Autodesk Inventor part; units mm, degrees
ref_plane "YZ Plane" through (0, 0, 0) normal (1, 0, 0) x (0, 1, 0)
ref_plane "XZ Plane" through (0, 0, 0) normal (0, 1, 0) x (-1, 0, 0)
ref_plane "XY Plane" through (0, 0, 0) normal (0, 0, 1) x (1, 0, 0)
sketch "Sketch1" plane through (0, 0, 0) normal (0, 1, 0) x (-1, 0, 0)
  line L0 (22.352, 6.35) -> (-46.355, 6.35)
  line L1 (-46.355, 6.35) -> (-46.355, -6.35)
  line L2 (-46.355, -6.35) -> (22.352, -6.35)
  line L3 (22.352, -6.35) -> (22.352, 6.35)
  line L4 (-2.3114, -2.3114) -> (2.3114, -2.3114)
  line L5 (2.3114, -2.3114) -> (2.3114, 2.3114)
  line L6 (2.3114, 2.3114) -> (-2.3114, 2.3114)
  line L7 (-2.3114, 2.3114) -> (-2.3114, -2.3114)
  line L8 (-2.3114, -2.3114) -> (2.3114, 2.3114) construction
  line L9 (2.3114, -2.3114) -> (-2.3114, 2.3114) construction
  line L10 (-10.3886, 2.3114) -> (-15.0114, 2.3114)
  line L11 (-15.0114, 2.3114) -> (-15.0114, -2.3114)
  line L12 (-15.0114, -2.3114) -> (-10.3886, -2.3114)
  line L13 (-10.3886, -2.3114) -> (-10.3886, 2.3114)
  line L14 (-10.3886, 2.3114) -> (-15.0114, -2.3114) construction
  line L15 (-15.0114, 2.3114) -> (-10.3886, -2.3114) construction
  line L16 (-23.0886, 2.3114) -> (-27.7114, 2.3114)
  line L17 (-27.7114, 2.3114) -> (-27.7114, -2.3114)
  line L18 (-27.7114, -2.3114) -> (-23.0886, -2.3114)
  line L19 (-23.0886, -2.3114) -> (-23.0886, 2.3114)
  line L20 (-23.0886, 2.3114) -> (-27.7114, -2.3114) construction
  line L21 (-27.7114, 2.3114) -> (-23.0886, -2.3114) construction
  point P0 (0, 0)
  point P1 (-12.7, 0)
  point P2 (-25.4, 0)
  dimension "d0" = 68.707
  dimension "d1" = 12.7
  dimension "d2" = 4.6228
  dimension "d3" = 4.6228
  dimension "d4" = 4.6228
  dimension "d5" = 4.6228
  dimension "d6" = 12.7
  dimension "d7" = 12.7
  dimension "d8" = 6.35
  dimension "d9" = 22.352
extrude "Extrusion1" add sketch "Sketch1" along normal blind 1.1684
sketch "Sketch2" plane through (0, 1.1684, 0) normal (0, 1, 0) x (1, 0, 0)
  line L0 (-22.352, 6.35) -> (-22.352, -6.35)
  circle A0 centre (-16.002, 0) radius 4.0259
  point P0 (0, 0)
  dimension "d12" = 6.35
  dimension "d13" = 8.0518
extrude "Extrusion2" add sketch "Sketch2" along normal blind 6.8326
sketch "Sketch3" plane through (-16.002, 8.001, 0) normal (0, 1, 0) x (1, 0, 0)
  circle A0 centre (0, 0) radius 2.8575
  point P0 (16.002, 0)
  dimension "d16" = 5.715
extrude "Extrusion3" cut sketch "Sketch3" against normal blind 0.7874
sketch "Sketch4" plane through (0, 0, 0) normal (0, -1, 0) x (1, 0, 0)
  circle A0 centre (-16.002, 0) radius 2.8575
  circle A1 centre (-16.002, 0) radius 2.8575
  point P0 (0, 0)
extrude "Extrusion4" cut sketch "Sketch4" against normal blind 0.7874
sketch "Sketch5" plane through (-16.002, 7.2136, 0) normal (0, 1, 0) x (1, 0, 0)
  circle A0 centre (0, 0) radius 2.4511
  point P0 (16.002, 0)
  dimension "d21" = 4.9022
extrude "Extrusion5" cut sketch "Sketch5" against normal through all
sketch "Sketch6" plane through (0, 1.1684, 0) normal (0, 1, 0) x (1, 0, 0)
  line L0 (46.355, -6.35) -> (46.355, 6.35)
  circle A0 centre (40.005, 0) radius 4.0259
  point P0 (0, 0)
  dimension "d24" = 6.35
  dimension "d25" = 8.0518
extrude "Extrusion6" add sketch "Sketch6" along normal blind 6.8326
sketch "Sketch7" plane through (40.005, 8.001, 0) normal (0, 1, 0) x (1, 0, 0)
  circle A0 centre (0, 0) radius 2.8575
  point P0 (-40.005, 0)
  dimension "d28" = 5.715
extrude "Extrusion7" cut sketch "Sketch7" against normal blind 0.7874
sketch "Sketch8" plane through (0, 0, 0) normal (0, -1, 0) x (1, 0, 0)
  circle A0 centre (40.005, 0) radius 2.8575
  circle A1 centre (40.005, 0) radius 2.8575
  point P0 (0, 0)
extrude "Extrusion8" cut sketch "Sketch8" against normal blind 0.7874
sketch "Sketch9" plane through (40.005, 7.2136, 0) normal (0, 1, 0) x (1, 0, 0)
  circle A0 centre (0, 0) radius 2.4511
  point P0 (-40.005, 0)
  dimension "d33" = 4.9022
extrude "Extrusion9" cut sketch "Sketch9" against normal through all
properties part number "VexLegoMount"
The model under review builds one solid part; all positions refer to its coordinate system, in mm. A direction names the side the tool comes from. Round coordinates to 2 decimals unless told otherwise and drop trailing zeros. Loops run counter-clockwise (first coordinate to the right, second up) from the corner with the lowest first, then second, coordinate; pieces in that order, holes last. Notation, with made-up numbers: M 2,-14.75 L 11,-14.75 A31 cw 11,21.25 Z; hole C 49.5,56 d3. An arc over 180 degrees is marked long. Answer as CSV lines item,"result". Start each with the question number.
Item 1: Insertion check: P1, Ø2, axis at y = 6, z = -2, coming from the -X side; P2, Ø3, axis at y = 4.5, z = 3, coming from the -X side. Each pin has a flat end and moves straight along its axis. Give the tip position at first contact, or say it passes through.
Item 2: Mouldability with a two-part tool opening along X and no side actions: class faces 4 (the face through (42.73, 0.39, 0.86)), 5 (the face through (46.355, 1, 0)), 6 (the face through (12, 0, -3)) as released by +X, released by -X, zero draft, split by the parting line, or undercut.
Item 3: Consider section C-C (x = -8.5). Write out the cut boundary in (y, z), then the cut area to 3 significant figures.
Item 4: Consider section D-D (z = 5.25). Write out the cut boundary in (x, y) (3 decimals).
Item 5: Wall thickness on line 1 (X direction, y = 3.25, z = 0.25); line 2 (X direction, y = 4, z = 0); line 3 (Z direction, x = -16, y = 4.75): over which ranges is each line inside the solid? List them lowest first. Write a range as [from, to].
Item 6: For faces 1 (the face through (35.983, 4.537, 0.177)), 2 (the face through (12, 1, 6.35)), 3 (the face through (2.311, 1, 0)), list the 3-axis set-ups (+Z, -Z, +X, -X, +Y, -Y) from which the entire face can be reached by the end or side of a thin tool; tool diameter is ignored.
Item 7: Consider section B-B (z = 0). State how many separate pieces and enclosed holes the cut face has, then the cut area to 3 significant figures.
Item 8: Consider section A-A (y = 6). Write out the cut boundary in (x, z) (3 decimals), then the cut area to 3 significant figures.
Answer:
1,P1,"stops at x = -19.9"
1,P2,"stops at x = -19.74"
2,face 4,"undercut"
2,face 5,"released by +X"
2,face 6,"zero draft"
3,outline,"M 0,-6.35 L 1.17,-6.35 L 1.17,6.35 L 0,6.35 Z"
3,area,"14.8 mm^2"
4,outline,"M -22.352,0 L 46.355,0 L 46.355,1.168 L -22.352,1.168 Z"
5,line 1,"x = [-20.02, -18.44], [-13.56, -11.98], [35.99, 37.57], [42.44, 44.02]"
5,line 2,"x = [-20.03, -18.45], [-13.55, -11.98], [35.98, 37.55], [42.46, 44.03]"
5,line 3,"z = [-4.03, -2.45], [2.45, 4.03]"
6,face 1,"+Y"
6,face 2,"+Z, +X, -X, +Y, -Y"
6,face 3,"+Y, -Y"
7,separate pieces,"6"
7,enclosed holes,"0"
7,area,"93.1 mm^2"
8,outline,"C -16.002,0 d8.052; C 40.005,0 d8.052; hole C -16.002,0 d4.902; hole C 40.005,0 d4.902"
8,area,"64.1 mm^2"
